Design review of the part built by this model. Coordinates are the model's own, in mm. Coordinates: 2 decimals unless noted, no trailing zeros. Loops run counter-clockwise (first coordinate to the right, second up) from the corner with the lowest first, then second, coordinate; pieces in that order, holes last. Notation, with made-up numbers: (74, 38.5) - (93, 38.5) arc R38 ccw to (93, 77.5) - close; hole circle Ø11 at (50, 89.25). An arc over 180 degrees is marked (long way). Return JSON: item names as keys, results as strings. Group by question number.
from build123d import *

# Parameters (mm, degrees)
SKETCH1_R                = 12.6746
BOSS_EXTRUDE1_DEPTH      = 1.016
BOSS_EXTRUDE1_DEPTH_BACK = 3.048
SKETCH3_W                = 1.6002
SKETCH3_H                = 2.499999953
CIRPATTERN1_COUNT        = 4


with BuildPart() as part:
    # Sketch1 → Boss-Extrude1 (new body, two sides)
    with BuildSketch(Plane.XY) as boss_extrude1_sk:
        with BuildLine():
            ThreePointArc((-5.461088217, 15.9766), (-11.938911845, 11.938911845), (-15.9766, 5.461088217))
            Line((-15.9766, 5.461088217), (-15.9766, -5.461088217))
            ThreePointArc((-15.9766, -5.461088217), (-11.938911845, -11.938911845), (-5.461088217, -15.9766))
            Line((-5.461088217, -15.9766), (5.461088217, -15.9766))
            ThreePointArc((5.461088217, -15.9766), (11.938911845, -11.938911845), (15.9766, -5.461088217))
            Line((15.9766, -5.461088217), (15.9766, 5.461088217))
            ThreePointArc((15.9766, 5.461088217), (11.938911845, 11.938911845), (5.461088217, 15.9766))
            Line((5.461088217, 15.9766), (-5.461088217, 15.9766))
        make_face()
        Circle(SKETCH1_R, mode=Mode.SUBTRACT)
    extrude(amount=BOSS_EXTRUDE1_DEPTH)
    extrude(boss_extrude1_sk.sketch, amount=-BOSS_EXTRUDE1_DEPTH_BACK)

    # Sketch3 → Cut-Revolve2 (revolve, cut)
    with BuildSketch(Plane.XY):
        with Locations((-14.4907, -1.249999977)):
            Rectangle(SKETCH3_W, SKETCH3_H)
    cut_revolve2 = revolve(axis=Axis((-13.6906, 0, 0), (-1, 0, 0)), mode=Mode.SUBTRACT)

    # CirPattern1: Cut-Revolve2 ×4 about axis
    cirpattern1_axis = Axis((0, 0, 0), (0, 0, 1))
    for i in range(1, CIRPATTERN1_COUNT):
        add(cut_revolve2.rotate(cirpattern1_axis, i * 360 / CIRPATTERN1_COUNT), mode=Mode.SUBTRACT)


solid = part.part
Item 1: Add section A-A (y = 0). State the section outline as (x, z) points.
Item 2: Add section D-D (x = 8). State the section outline as (y, z) points.
Item 3: Add section C-C (z = -1.1). State the section outline as (x, y) points (3 decimals).
Item 4: To check wall thickness, follow line 1 (Y direction, x = 0, z = -1.5); line 2 (Z direction, x = 0, y = 14.6); line 3 (Y direction, x = 5, z = -1.45). State the ranges of each line that lie inside material, in increasing order. Write a range as from..to.
Item 5: Draft analysis for pull direction X (two halves, no side actions). For faces 1 (the face through (12.015, 11.862, -0.988)), 2 (the face through (13.691, 0, 0)), 3 (the face through (0, -15.977, -1)), state which applies: pulls with the +X half, pulls with the -X half, needs draft (parallel to the pull), parting line crosses it, or undercut.
Answers below:
{
 "1": {"outline": "(-15.98, -3.05) - (-12.67, -3.05) - (-12.67, 1.02) - (-13.69, 1.02) - (-13.69, -2.5) - (-15.29, -2.5) - (-15.29, 1.02) - (-15.98, 1.02) - close; (12.67, -3.05) - (15.98, -3.05) - (15.98, 1.02) - (15.29, 1.02) - (15.29, -2.5) - (13.69, -2.5) - (13.69, 1.02) - (12.67, 1.02) - close"},
 "2": {"outline": "(-14.87, -3.05) - (-9.83, -3.05) - (-9.83, 1.02) - (-14.87, 1.02) - close; (9.83, -3.05) - (14.87, -3.05) - (14.87, 1.02) - (9.83, 1.02) - close"},
 "3": {"outline": "(-15.977, -5.461) arc R16.884 ccw to (-5.461, -15.977) - (5.461, -15.977) arc R16.884 ccw to (15.977, -5.461) - (15.977, 5.461) arc R16.884 ccw to (5.461, 15.977) - (-5.461, 15.977) arc R16.884 ccw to (-15.977, 5.461) - close; hole (-15.291, -2.245) - (-13.691, -2.245) - (-13.691, 2.245) - (-15.291, 2.245) - close; hole circle Ø25.349 at (0, 0); hole (-2.245, -15.291) - (2.245, -15.291) - (2.245, -13.691) - (-2.245, -13.691) - close; hole (-2.245, 13.691) - (2.245, 13.691) - (2.245, 15.291) - (-2.245, 15.291) - close; hole (13.691, -2.245) - (15.291, -2.245) - (15.291, 2.245) - (13.691, 2.245) - close"},
 "4": {"line 1": "y = -15.98..-15.29, -13.69..-12.67, 12.67..13.69, 15.29..15.98", "line 2": "z = -3.05..-2.5", "line 3": "y = -15.98..-11.65, 11.65..15.98"},
 "5": {"face 1": "pulls with the +X half", "face 2": "undercut", "face 3": "needs draft"}
}
